For this review, use the dimensioned drawing (mm, ordinates from the lowest corner) and the shaded views. A direction names the side the tool comes from. Round coordinates to 2 decimals unless told otherwise and drop trailing zeros. Order: outer loops, then holes, each group sorted by start corner. A loop starts at its lowest first (then second) coordinate and runs counter-clockwise, first axis right, second up. Notation, with made-up numbers: M -36,34 L -30,34 A25 cw -30,63 Z; hole C 53,43.25 d5. An arc over 180 degrees is marked long. Put each result on its own line as item: value.
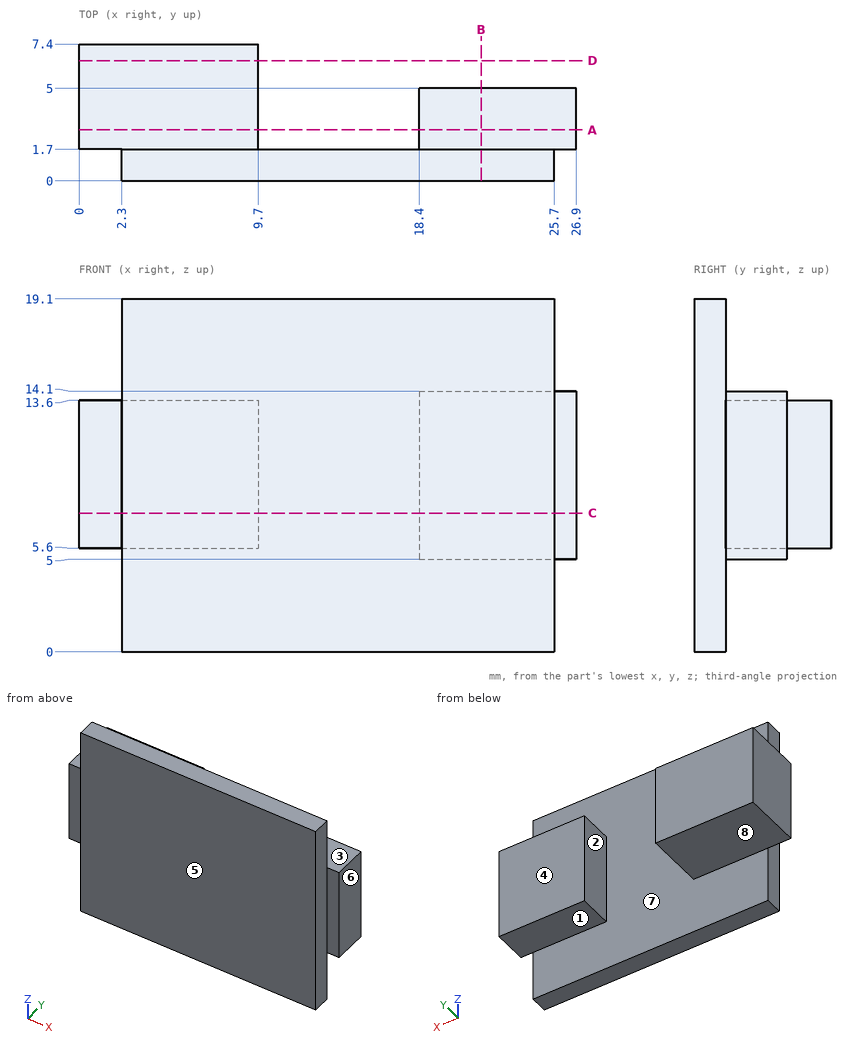
(1) For the marked faces 1, 2, 3, 4 and 5, list the 3-axis set-ups (+Z, -Z, +X, -X, +Y, -Y) from which the entire face can be reached by the end or side of a thin tool; tool diameter is ignored.
A:
face 1: -Z, +X, -X, +Y
face 2: +Z, -Z, +Y
face 3: +Z, +X, -X, +Y
face 4: +Z, -Z, +X, +Y
face 5: +Z, -Z, +X, -X, -Y
(2) Draft analysis for pull direction X (two halves, no side actions). For the marked faces 6, 7 and 8, state which applies: released by +X, released by -X, zero draft, split by the parting line, or undercut.
A:
face 6: released by +X
face 7: undercut
face 8: zero draft
(3) Add section C-C on z = 7.5. Give the boundary of the cut face in (x, y), then the cut area to 3 significant figures.
A:
outline: M 0,1.7 L 2.3,1.7 L 2.3,0 L 25.7,0 L 25.7,1.7 L 26.9,1.7 L 26.9,5 L 18.4,5 L 18.4,1.7 L 9.7,1.7 L 9.7,7.4 L 0,7.4 Z
area: 123 mm2
(4) Add section D-D on y = 6.5. Give the boundary of the cut face in (x, z).
A:
outline: M 0,5.6 L 9.7,5.6 L 9.7,13.6 L 0,13.6 Z
(5) To check wall thickness, follow L1, parallel to X at y = 2.5, z = 13; L2, parallel to Y at x = 19.5, z = 2.25; L3, parallel to Y at x = 19.5, z = 14. State the ranges of each line that lie inside material, in increasing order.
A:
L1: x = 0 to 9.7, 18.4 to 26.9
L2: y = 0 to 1.7
L3: y = 0 to 5
(6) Add section B-B on x = 21.75. Give the boundary of the cut face in (y, z), then the cut area to 3 significant figures.
A:
outline: M 0,0 L 1.7,0 L 1.7,5 L 5,5 L 5,14.1 L 1.7,14.1 L 1.7,19.1 L 0,19.1 Z
area: 62.5 mm2
(7) Add section A-A on y = 2.75. Give the boundary of the cut face in (x, z).
A:
outline: M 0,5.6 L 9.7,5.6 L 9.7,13.6 L 0,13.6 Z; M 18.4,5 L 26.9,5 L 26.9,14.1 L 18.4,14.1 Z
(8) Insertion check: pin 1 Ø2.5 at (x, y) = (24.5, 3.5) entering from -Z; pin 2 Ø10 at (x, z) = (17.5, 5.5) entering from +Y; pin 3 Ø4 at (x, y) = (22.5, 4) entering from +Z; pin 4 Ø1.6 at (y, z) = (4, 11) entering from -X. Each pin has a flat end and moves straight along its axis. Give the tip position at first contact, or say it passes through.
A:
pin 1: stops at z = 5
pin 2: stops at y = 5
pin 3: stops at z = 14.1
pin 4: stops at x = 0
